from build123d import *

# Parameters (mm, degrees)
SKETCH_1_R          = 6
EXTRUDE_1_DEPTH     = 105
CUT_EXTRUDE_START   = -5.8
SKETCH_2_R          = 6
SKETCH_2_R_2        = 5
CUT_EXTRUDE_1_DEPTH = 5.8


with BuildPart() as part:
    # ｽｹｯﾁ1 → ﾎﾞｽ - 押し出し1 (new, symmetric)
    with BuildSketch(Plane.XY):
        Circle(SKETCH_1_R)
    extrude(amount=EXTRUDE_1_DEPTH, both=True)

    # ｽｹｯﾁ2 → ｶｯﾄ - 押し出し1 (cut)
    with BuildSketch(Plane(origin=(0, 0, -105), x_dir=(-1, 0, 0), z_dir=(0, 0, -1)).offset(CUT_EXTRUDE_START)):
        Circle(SKETCH_2_R)
        Circle(SKETCH_2_R_2, mode=Mode.SUBTRACT)
    cut_extrude_1 = extrude(amount=CUT_EXTRUDE_1_DEPTH, mode=Mode.SUBTRACT)

    # ﾐﾗｰ1: ｶｯﾄ - 押し出し1 across plane
    add(cut_extrude_1.mirror(Plane.XY), mode=Mode.SUBTRACT)


solid = part.part
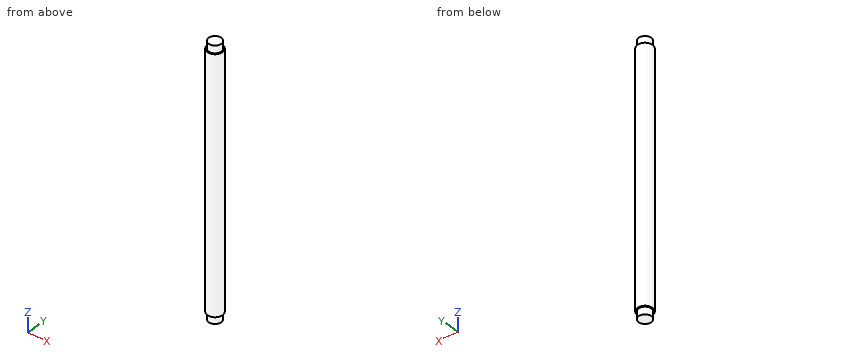
Input: part model. Units: mm. Frame: model coordinates. Round coordinates to 2 decimals unless told otherwise and drop trailing zeros. Loops run counter-clockwise (first coordinate to the right, second up) from the corner with the lowest first, then second, coordinate; pieces in that order, holes last. Notation, with made-up numbers: (73.25, 3.5) -> (116.25, 3.5) arc R34 ccw to (116.25, 35.5) -> close; hole circle Ø4 at (27, 38.5). An arc over 180 degrees is marked (long way). Answer as a JSON object with one key per item and string values. Group by question number.
1) Section query B-B on x = -1.75. Output: boundary loops of the cut face in (y, z).
2) Section query C-C on y = 2. Output: boundary loops of the cut face in (x, z).
3) Pin query (flat end, axial travel): pin 1 (1 mm diameter, centred on x = -5, y = 4.5, fed in from +Z); pin 2 (5 mm diameter, centred on y = 1, z = 52.5, fed in from -X); pin 3 (5 mm diameter, centred on x = -4, z = -50, fed in from -Y); pin 4 (1 mm diameter, centred on y = 3.5, z = -67, fed in from -X). Return the tip coordinate at first contact, or that it passes through.
4) Ray query, L1, parallel to Z at x = -5, y = 2.75; L2, parallel to Y at x = -3.25, z = -59.5; L3, parallel to Y at x = -0.25, z = 13. Return the intervals inside material, ascending.
5) Section query A-A on z = 88. Output: boundary loops of the cut face in (x, y).
Reply:
{
 "1": {"outline": "(-5.74, -99.2) -> (-4.68, -99.2) -> (-4.68, -105) -> (4.68, -105) -> (4.68, -99.2) -> (5.74, -99.2) -> (5.74, 99.2) -> (4.68, 99.2) -> (4.68, 105) -> (-4.68, 105) -> (-4.68, 99.2) -> (-5.74, 99.2) -> close"},
 "2": {"outline": "(-5.66, -99.2) -> (-4.58, -99.2) -> (-4.58, -105) -> (4.58, -105) -> (4.58, -99.2) -> (5.66, -99.2) -> (5.66, 99.2) -> (4.58, 99.2) -> (4.58, 105) -> (-4.58, 105) -> (-4.58, 99.2) -> (-5.66, 99.2) -> close"},
 "3": {"pin 1": "passes through", "pin 2": "stops at x = -6", "pin 3": "stops at y = -5.81", "pin 4": "stops at x = -5.2"},
 "4": {"L1": "z = -99.2 to 99.2", "L2": "y = -5.04 to 5.04", "L3": "y = -5.99 to 5.99"},
 "5": {"outline": "circle Ø12 at (0, 0)"}
}
